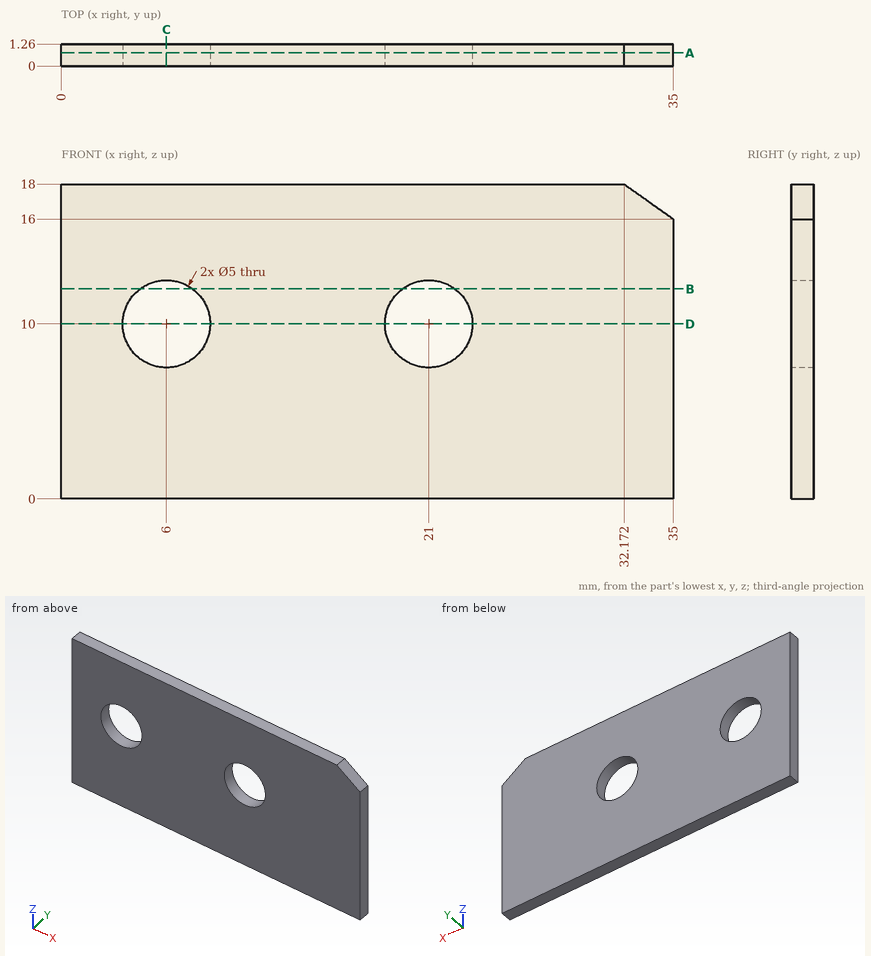
Can you work these out from the drawing? Everything is in mm from the part's minimum corner. Round coordinates to 2 decimals unless told otherwise and drop trailing zeros. Loops run counter-clockwise (first coordinate to the right, second up) from the corner with the lowest first, then second, coordinate; pieces in that order, holes last. Notation, with made-up numbers: (85, -17) - (90, -17) arc R18 ccw to (90, 13) - close; hole circle Ø1 at (-12, 7). An arc over 180 degrees is marked (long way). One line per question, with ' | ' between items. Start each with the question number.
Q1. I want a section at B-B (z = 12). Write out the boundary of the cut face in (x, y).
Q2. I want a section at C-C (x = 6). Write out the boundary of the cut face in (y, z).
Q3. I want a section at D-D (z = 10). Write out the boundary of the cut face in (x, y), then the cut area to 3 significant figures.
Q4. I want a section at A-A (y = 0.75). Write out the boundary of the cut face in (x, z).
Q5. Please list where these lines run through material, in increasing order: line 1 (X direction, y = 0.5, z = 10); line 2 (X direction, y = 0.85, z = 8.75) (1 decimal); line 3 (Z direction, x = 19.5, y = 1.15). Write a range as [from, to].
Response values:
1) outline: (0, 0) - (4.5, 0) - (4.5, 1.26) - (0, 1.26) - close; (7.5, 0) - (19.5, 0) - (19.5, 1.26) - (7.5, 1.26) - close; (22.5, 0) - (35, 0) - (35, 1.26) - (22.5, 1.26) - close
2) outline: (0, 0) - (1.26, 0) - (1.26, 7.5) - (0, 7.5) - close; (0, 12.5) - (1.26, 12.5) - (1.26, 18) - (0, 18) - close
3) outline: (0, 0) - (3.5, 0) - (3.5, 1.26) - (0, 1.26) - close; (8.5, 0) - (18.5, 0) - (18.5, 1.26) - (8.5, 1.26) - close; (23.5, 0) - (35, 0) - (35, 1.26) - (23.5, 1.26) - close | area: 31.5 mm²
4) outline: (0, 0) - (35, 0) - (35, 16) - (32.17, 18) - (0, 18) - close; hole circle Ø5 at (6, 10); hole circle Ø5 at (21, 10)
5) line 1: x = [0, 3.5], [8.5, 18.5], [23.5, 35] | line 2: x = [0, 3.8], [8.2, 18.8], [23.2, 35] | line 3: z = [0, 8], [12, 18]
